Check sheet for the modelled part. Datum: model origin and axes. Units: mm. Face numbers are marked on the shaded views. A direction names the side the tool comes from. Round coordinates to 2 decimals unless told otherwise and drop trailing zeros. Write each loop counter-clockwise with the first axis right and the second up, starting at its lowest first coordinate (ties: lowest second). Pieces come first, ordered by that corner, then holes. Notation, with made-up numbers: (-39, -27.75) -> (-9, -27.75) arc R26 ccw to (-9, 11.25) -> close; hole circle Ø11 at (-38.75, 6.5). An arc over 180 degrees is marked (long way). One line per item, written item: value.
from build123d import *

# Parameters (mm, degrees)
SKETCH1_R           = 1.1
SKETCH1_R_2         = 1.6
BOSS_EXTRUDE1_DEPTH = 15
CUT_EXTRUDE1_DEPTH  = 15
SKETCH4_W           = 1.8
SKETCH4_H           = 0.5
BOSS_EXTRUDE2_DEPTH = 15


with BuildPart() as part:
    # Sketch1 → Boss-Extrude1 (new body)
    with BuildSketch(Plane.XY):
        with BuildLine():
            Line((-1.61243197, 5.01974999), (-5.34022711, 2.600340269))
            ThreePointArc((-5.34022711, 2.600340269), (-6.625018483, -0.880041239), (-3.652556975, -3.1))
            Line((-3.652556975, -3.1), (4.395993446, -3.201847309))
            ThreePointArc((4.395993446, -3.201847309), (7.362670385, -1.001195929), (6.117333323, 2.476328214))
            Line((6.117333323, 2.476328214), (2.346418367, 4.994010285))
            ThreePointArc((2.346418367, 4.994010285), (0.370849058, 5.59992391), (-1.61243197, 5.01974999))
        make_face()
        with Locations((4.347443025, 0)):
            Circle(SKETCH1_R, mode=Mode.SUBTRACT)
        with Locations((0.347443025, 2)):
            Circle(SKETCH1_R_2, mode=Mode.SUBTRACT)
        with Locations((-3.652556975, 0)):
            Circle(SKETCH1_R, mode=Mode.SUBTRACT)
    extrude(amount=BOSS_EXTRUDE1_DEPTH)

    # Sketch3 → Cut-Extrude1 (cut)
    with BuildSketch(Plane.XY.offset(15)):
        with BuildLine():
            Line((-3.652556975, -3.1), (-3.652556975, -1.1))
            ThreePointArc((-3.652556975, -1.1), (-4.430374434, -0.777817459), (-4.752556975, 0))
            Line((-4.752556975, 0), (-6.752556975, 0))
            ThreePointArc((-6.752556975, 0), (-5.844587997, -2.192031022), (-3.652556975, -3.1))
        make_face()
        with BuildLine():
            Line((3.247443025, 0), (-2.552556975, 0))
            ThreePointArc((-2.552556975, 0), (-2.874739516, -0.777817459), (-3.652556975, -1.1))
            Line((-3.652556975, -1.1), (-3.652556975, -3.1))
            Line((-3.652556975, -3.1), (4.395993446, -3.201847309))
            ThreePointArc((4.395993446, -3.201847309), (6.623741934, -2.257569154), (7.49431995, 0))
            Line((7.49431995, 0), (5.447443025, 0))
            ThreePointArc((5.447443025, 0), (4.347443025, -1.1), (3.247443025, 0))
        make_face()
        with BuildLine():
            Line((-3.652556975, -4.774585684), (-3.652556975, -3.1))
            ThreePointArc((-3.652556975, -3.1), (-5.844587997, -2.192031022), (-6.752556975, 0))
            Line((-6.752556975, 0), (-12.259555469, 0))
            Line((-12.259555469, 0), (-12.259555469, -4.774585684))
            Line((-12.259555469, -4.774585684), (-3.652556975, -4.774585684))
        make_face()
        with BuildLine():
            Line((4.395993446, -3.201847309), (-3.652556975, -3.1))
            Line((-3.652556975, -3.1), (-3.652556975, -4.774585684))
            Line((-3.652556975, -4.774585684), (12.655202498, -4.774585684))
            Line((12.655202498, -4.774585684), (12.655202498, 0))
            Line((12.655202498, 0), (7.49431995, 0))
            ThreePointArc((7.49431995, 0), (6.623741934, -2.257569154), (4.395993446, -3.201847309))
        make_face()
    extrude(amount=-CUT_EXTRUDE1_DEPTH, mode=Mode.SUBTRACT)

    # Sketch4 → Boss-Extrude2 (add)
    with BuildSketch(Plane.XY.offset(15)):
        with Locations((0.347443025, -0.25)):
            Rectangle(SKETCH4_W, SKETCH4_H)
    extrude(amount=-BOSS_EXTRUDE2_DEPTH)


solid = part.part
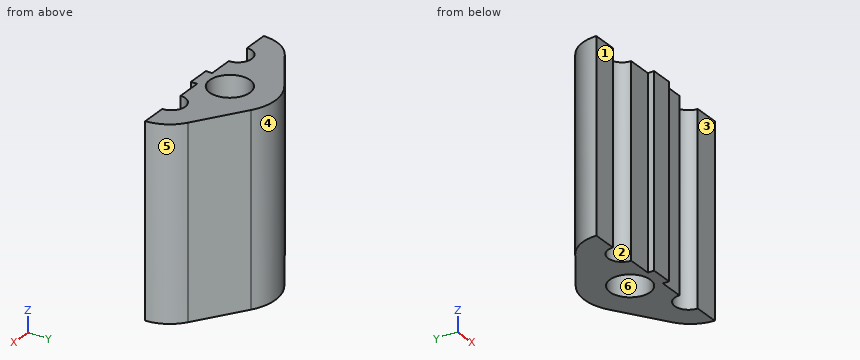
Item 1: Sectioned sample at D-D on x = -2.25. Enter the section's corners in (y, z).
Answer:
outline: (0, 0) -> (4.61, 0) -> (4.61, 15) -> (0, 15) -> close
Item 2: Sectioned sample at A-A on y = 0.75. Enter the section's corners in (x, z).
Answer:
outline: (-6.66, 0) -> (-4.46, 0) -> (-4.46, 15) -> (-6.66, 15) -> close; (-2.85, 0) -> (-0.65, 0) -> (-0.65, 15) -> (-2.85, 15) -> close; (1.35, 0) -> (3.54, 0) -> (3.54, 15) -> (1.35, 15) -> close; (5.15, 0) -> (7.38, 0) -> (7.38, 15) -> (5.15, 15) -> close
Item 3: Sectioned sample at B-B on x = 0. Enter the section's corners in (y, z), and give its area (3 significant figures).
Answer:
outline: (-0.5, 0) -> (0.44, 0) -> (0.44, 15) -> (-0.5, 15) -> close; (3.56, 0) -> (5.58, 0) -> (5.58, 15) -> (3.56, 15) -> close
area: 44.4 mm^2
Item 4: Sectioned sample at C-C on y = 3.25. Enter the section's corners in (x, z), and give its area (3 significant figures).
Answer:
outline: (-4.34, 0) -> (-0.65, 0) -> (-0.65, 15) -> (-4.34, 15) -> close; (1.35, 0) -> (4.96, 0) -> (4.96, 15) -> (1.35, 15) -> close
area: 110 mm^2
Item 5: Tool access check on the marked faces 1, 2 and 3. Record the directions out of +Z, -Z, +X, -X, +Y, -Y that give a thin tool (end or side, any length) a straight path to the whole face; none if there is none.
Answer:
face 1: +Z, -Z, -X, -Y
face 2: +Z, -Z, -Y
face 3: +Z, -Z, +X, -Y
Item 6: Mould release check, pull along X, two halves, no side actions. Record for the marked faces 4, 5 and 6: pulls with the +X half, pulls with the -X half, needs draft (parallel to the pull), parting line crosses it, or undercut.
Answer:
face 4: parting line crosses it
face 5: pulls with the +X half
face 6: undercut
Item 7: Thickness scan on line 1 (X direction, y = 2.75, z = 11.75); line 2 (Y direction, x = -0.5, z = 4.5); line 3 (Y direction, x = 0, z = 12). Record the ranges inside material, lowest first.
Answer:
line 1: x = -5.11 to -1.07, 1.76 to 5.71
line 2: y = -0.5 to 0.64, 3.36 to 5.5
line 3: y = -0.5 to 0.44, 3.56 to 5.58
Item 8: Depth check by flat-ended pin: P1, Ø1.6, axis at x = 6, z = 9.5, coming from the -Y side; P2, Ø0.6, axis at y = -0.5, z = 6.5, coming from the +X side; P3, Ø3.5, axis at x = 0.35, y = 2, coming from the -Z side; P4, Ø1, axis at x = -0.5, y = 1.5, coming from the -Z side. Enter the tip coordinate at first touch or a pass-through.
Answer:
P1: stops at y = 0
P2: stops at x = 1.25
P3: stops at z = 0
P4: passes through
